```python
from build123d import *

# Parameters (mm, degrees)
SKETCH2_W           = 100
SKETCH2_H           = 100
BOSS_EXTRUDE2_DEPTH = 100
SKETCH4_W           = 88.827102195
SKETCH4_H           = 58.821478126
CUT_EXTRUDE1_DEPTH  = 100
SKETCH6_W           = 88.733960409
SKETCH6_H           = 88.503004296
BOSS_EXTRUDE3_DEPTH = 3


with BuildPart() as part:
    # Sketch2 → Boss-Extrude2 (new body)
    with BuildSketch(Plane.XY):
        with Locations((0, 50)):
            Rectangle(SKETCH2_W, SKETCH2_H)
    extrude(amount=BOSS_EXTRUDE2_DEPTH)

    # Sketch4 → Cut-Extrude1 (cut)
    with BuildSketch(Plane(origin=(0, 100, 0), x_dir=(1, 0, 0), z_dir=(0, 1, 0))):
        with Locations((5.586448902, -50)):
            Rectangle(SKETCH4_W, SKETCH4_H)
        with BuildLine():
            Line((-38.827102195, -88), (-38.827102195, -100))
            Line((-38.827102195, -100), (47, -100))
            ThreePointArc((47, -100), (39.928932188, -97.071067812), (37, -90))
            Line((37, -90), (37, -88))
            Line((37, -88), (-38.827102195, -88))
        make_face()
        with BuildLine():
            Line((47, 0), (-38.827102195, 0))
            Line((-38.827102195, 0), (-38.827102195, -12))
            Line((-38.827102195, -12), (37, -12))
            Line((37, -12), (37, -10))
            ThreePointArc((37, -10), (39.928932188, -2.928932188), (47, 0))
        make_face()
    extrude(amount=-CUT_EXTRUDE1_DEPTH, mode=Mode.SUBTRACT)

    # Sketch6 → Boss-Extrude3 (add)
    with BuildSketch(Plane.ZY.offset(50)):
        with Locations((49.115734201, 50.114251056)):
            Rectangle(SKETCH6_W, SKETCH6_H)
    extrude(amount=BOSS_EXTRUDE3_DEPTH)


solid = part.part
```
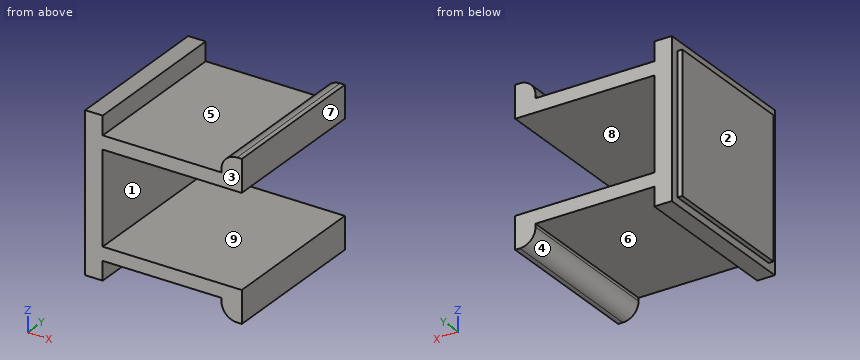
The model under review builds one solid part; all positions refer to its coordinate system, in mm. Face numbers are marked on the shaded views. A direction names the side the tool comes from. Give positions to 0.01 mm unless a question says otherwise; leave off trailing zeros. Write each loop counter-clockwise with the first axis right and the second up, starting at its lowest first coordinate (ties: lowest second). Pieces come first, ordered by that corner, then holes.
(1) For P1, Ø10, axis at x = 26, y = 16.5, coming from the +Z side; P2, Ø3.5, axis at x = -51, z = 64, coming from the -Y side; P3, Ø1.5, axis at x = -52, z = 60.5, coming from the +Y side; P4, Ø3.5, axis at x = -52, y = 30, coming from the -Z side, all flat-tipped, find the tip position at first contact; note any pin that passes through.
(2) The part is to be moulded in two halves that separate along Z. For the marked faces 6, 7, 8 and 9, say which applies: released by +Z, released by -Z, zero draft, split by the parting line, or undercut.
(3) Consider section C-C, the plane z = 42. Give the boundary of the cut face in (x, y).
(4) Tool access review of the marked faces 1, 2, 3, 4 and 5: name each direction out of +Z, -Z, +X, -X, +Y, -Y from which nothing blocks a thin tool from reaching the whole face with its end or side.
(5) To check wall thickness, follow L1, parallel to Z at x = 30.5, y = 83; L2, parallel to X at y = 83.5, z = 90.5; L3, parallel to X at y = 39.5, z = 37.5. State the ranges of each line that lie inside material, in increasing order.
(6) Consider section D-D, the plane x = 43.5. Give the boundary of the cut face in (y, z), and give its area (3 significant figures).
(7) Consider section A-A, the plane x = -10. Give the boundary of the cut face in (y, z).
(8) Consider section B-B, the plane y = 39.5. Give the boundary of the cut face in (x, z).
Returned:
1. P1: stops at z = 88
1. P2: stops at y = 0
1. P3: stops at y = 94.37
1. P4: stops at z = 4.75
2. face 6: released by -Z
2. face 7: zero draft
2. face 8: undercut
2. face 9: undercut
3. outline: (-53, 5.86) - (-50, 5.86) - (-50, 0) - (-38.83, 0) - (-38.83, 100) - (-50, 100) - (-50, 94.37) - (-53, 94.37) - close
4. face 1: +X, +Y, -Y
4. face 2: +Z, -Z, -X, +Y, -Y
4. face 3: +Z, -Z, +X, -X, -Y
4. face 4: -Z, +Y, -Y
4. face 5: +Z, +Y, -Y
5. L1: z = 12 to 20.59, 79.41 to 88
5. L2: x = -53 to -38.83, 37.01 to 50
5. L3: x = -53 to -38.83
6. outline: (0, 0.63) - (100, 0.63) - (100, 20.59) - (0, 20.59) - close; (0, 79.41) - (100, 79.41) - (100, 99.37) - (0, 99.37) - close
6. area: 3,990 mm2
7. outline: (0, 12) - (100, 12) - (100, 20.59) - (0, 20.59) - close; (0, 79.41) - (100, 79.41) - (100, 88) - (0, 88) - close
8. outline: (-53, 4.75) - (-50, 4.75) - (-50, 0) - (-38.83, 0) - (-38.83, 12) - (37, 12) - (37, 10) arc R10 ccw to (47, 0) - (50, 0) - (50, 20.59) - (-38.83, 20.59) - (-38.83, 79.41) - (50, 79.41) - (50, 100) - (47, 100) arc R10 ccw to (37, 90) - (37, 88) - (-38.83, 88) - (-38.83, 100) - (-50, 100) - (-50, 93.48) - (-53, 93.48) - close
